Study the drawing (mm; zero at the part's minimum x, y, z) and answer. A direction names the side the tool comes from. Coordinates: 2 decimals unless noted, no trailing zeros. Order: outer loops, then holes, each group sorted by start corner. A loop starts at its lowest first (then second) coordinate and runs counter-clockwise, first axis right, second up.
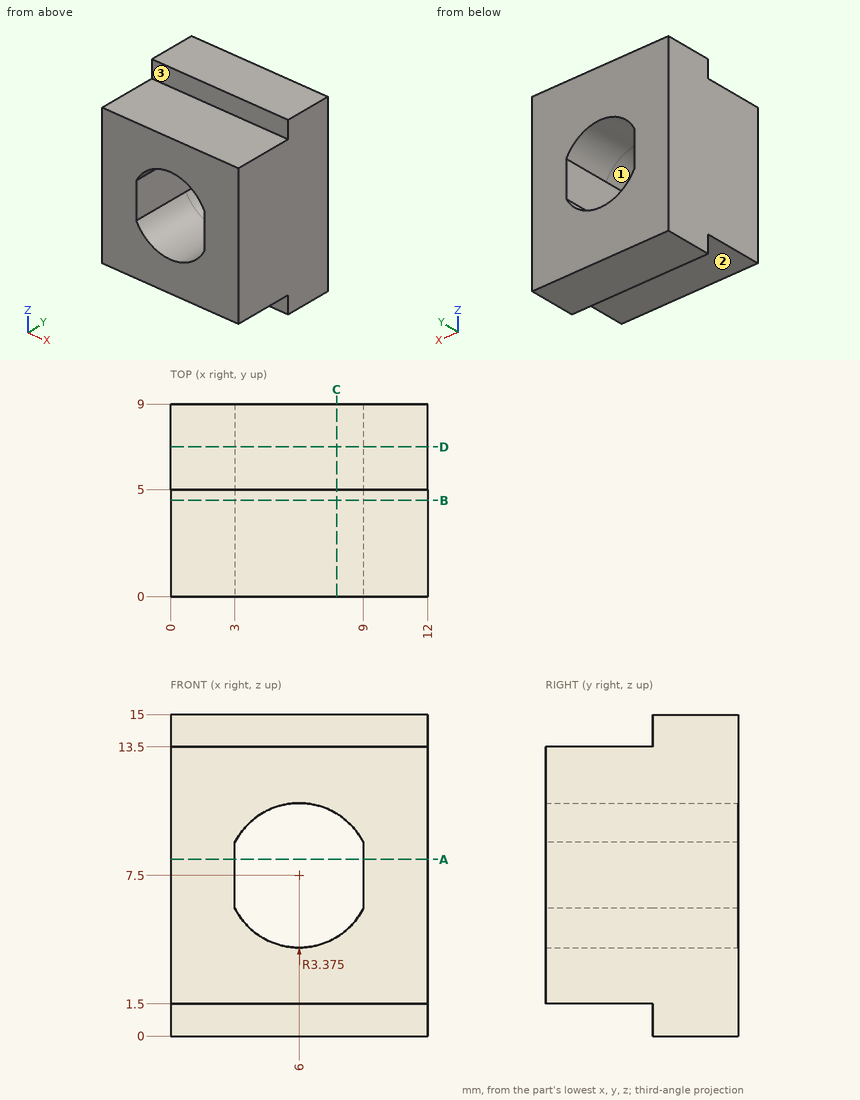
(1) Find section A-A on z = 8.25. Determine the outline of the cut face in (x, y).
(2) Find section D-D on y = 7. Determine the outline of the cut face in (x, z) (3 decimals), then the cut area to 3 significant figures.
(3) Find section B-B on y = 4.5. Determine the outline of the cut face in (x, z) (3 decimals), then the cut area to 3 significant figures.
(4) A tool of negligible diameter and unlimited length cuts with its end or side. For the marked faces 1, 2 and 3, from which of +Z, -Z, +X, -X, +Y, -Y can it reach the whole face along a straight path? Write none if from no direction.
(5) Given pin 1 Ø1.5 at (y, z) = (4.5, 5.5) entering from -X; pin 2 Ø4 at (x, y) = (5, 1.5) entering from -Z, each flat-ended and moving along its own axis, determine where each tip first touches the part or whether it passes through.
(6) Find section C-C on x = 7.75. Determine the outline of the cut face in (y, z), then the cut area to 3 significant figures.
(7) Find the intervals of material crossed by probe 1 along X at (y, z) = (8.5, 8); probe 2 along X at (y, z) = (3.5, 10.25); probe 3 along Y at (x, z) = (8.25, 13.75), in increasing order.
Resolved:
1. outline: (0, 0) - (3, 0) - (3, 9) - (0, 9) - close; (9, 0) - (12, 0) - (12, 9) - (9, 9) - close
2. outline: (0, 0) - (12, 0) - (12, 15) - (0, 15) - close; hole (3, 5.954) arc R3.375 ccw to (9, 5.954) - (9, 9.046) arc R3.375 ccw to (3, 9.046) - close
2. area: 146 mm2
3. outline: (0, 1.5) - (12, 1.5) - (12, 13.5) - (0, 13.5) - close; hole (3, 5.954) arc R3.375 ccw to (9, 5.954) - (9, 9.046) arc R3.375 ccw to (3, 9.046) - close
3. area: 110 mm2
4. face 1: +Y, -Y
4. face 2: -Z, +X, -X, -Y
4. face 3: +Z, +X, -X, -Y
5. pin 1: stops at x = 0
5. pin 2: stops at z = 1.5
6. outline: (0, 1.5) - (5, 1.5) - (5, 0) - (9, 0) - (9, 4.61) - (0, 4.61) - close; (0, 10.39) - (9, 10.39) - (9, 15) - (5, 15) - (5, 13.5) - (0, 13.5) - close
6. area: 68.1 mm2
7. probe 1: x = 0 to 3, 9 to 12
7. probe 2: x = 0 to 4.04, 7.96 to 12
7. probe 3: y = 5 to 9
